Verification items for the finished model (mm, model axes). Face numbers are marked on the shaded views. A direction names the side the tool comes from. Round coordinates to 2 decimals unless told otherwise and drop trailing zeros. Write each loop counter-clockwise with the first axis right and the second up, starting at its lowest first coordinate (ties: lowest second). Pieces come first, ordered by that corner, then holes.
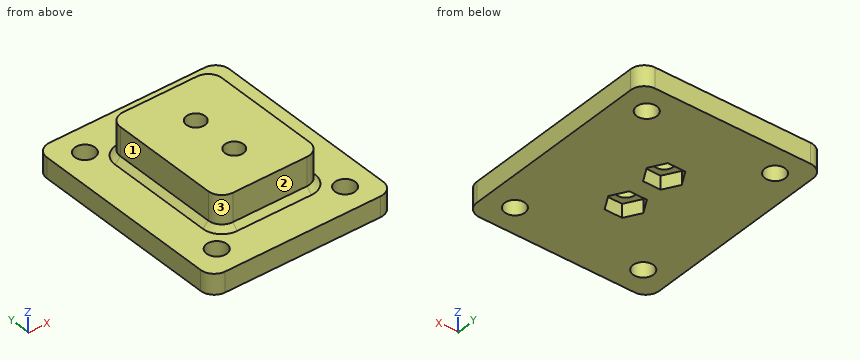
from build123d import *

# Parameters (mm, degrees)
F0_R     = 4.365625
F0_R_2   = 4.7625
F1_DEPTH = 9.525
F2_DEPTH = 25.4
F3_SIZE  = 2.54
F4_DEPTH = 6.35


with BuildPart() as f1:
    # F0 (on Top) → F1 (new body)
    with BuildSketch(Plane.XY):
        Polygon((-4.124446, -18.25625), (4.124446, -18.25625), (8.248892, -11.1125), (4.124446, -3.96875), (-4.124446, -3.96875), (-8.248892, -11.1125), align=None)
        with Locations((0, -11.1125)):
            Circle(F0_R, mode=Mode.SUBTRACT)
        with BuildLine():
            Line((17.4625, 31.75), (-17.4625, 31.75))
            ThreePointArc((-17.4625, 31.75), (-21.952628, 29.890128), (-23.8125, 25.4))
            Line((-23.8125, 25.4), (-23.8125, -25.4))
            ThreePointArc((-23.8125, -25.4), (-21.952628, -29.890128), (-17.4625, -31.75))
            Line((-17.4625, -31.75), (17.4625, -31.75))
            ThreePointArc((17.4625, -31.75), (21.952628, -29.890128), (23.8125, -25.4))
            Line((23.8125, -25.4), (23.8125, 25.4))
            ThreePointArc((23.8125, 25.4), (21.952628, 29.890128), (17.4625, 31.75))
        make_face()
        Polygon((8.248892, -11.1125), (4.124446, -18.25625), (-4.124446, -18.25625), (-8.248892, -11.1125), (-4.124446, -3.96875), (4.124446, -3.96875), align=None, mode=Mode.SUBTRACT)
        Polygon((-8.248892, 11.1125), (-4.124446, 18.25625), (4.124446, 18.25625), (8.248892, 11.1125), (4.124446, 3.96875), (-4.124446, 3.96875), align=None, mode=Mode.SUBTRACT)
        with BuildLine():
            Line((36.5125, 50.8), (-36.5125, 50.8))
            ThreePointArc((-36.5125, 50.8), (-41.002628, 48.940128), (-42.8625, 44.45))
            Line((-42.8625, 44.45), (-42.8625, -44.45))
            ThreePointArc((-42.8625, -44.45), (-41.002628, -48.940128), (-36.5125, -50.8))
            Line((-36.5125, -50.8), (36.5125, -50.8))
            ThreePointArc((36.5125, -50.8), (41.002628, -48.940128), (42.8625, -44.45))
            Line((42.8625, -44.45), (42.8625, 44.45))
            ThreePointArc((42.8625, 44.45), (41.002628, 48.940128), (36.5125, 50.8))
        make_face()
        with Locations((-30.1625, -38.1)):
            Circle(F0_R_2, mode=Mode.SUBTRACT)
        with Locations((30.1625, -38.1)):
            Circle(F0_R_2, mode=Mode.SUBTRACT)
        with BuildLine():
            ThreePointArc((-23.8125, 25.4), (-21.952628, 29.890128), (-17.4625, 31.75))
            Line((-17.4625, 31.75), (17.4625, 31.75))
            ThreePointArc((17.4625, 31.75), (21.952628, 29.890128), (23.8125, 25.4))
            Line((23.8125, 25.4), (23.8125, -25.4))
            ThreePointArc((23.8125, -25.4), (21.952628, -29.890128), (17.4625, -31.75))
            Line((17.4625, -31.75), (-17.4625, -31.75))
            ThreePointArc((-17.4625, -31.75), (-21.952628, -29.890128), (-23.8125, -25.4))
            Line((-23.8125, -25.4), (-23.8125, 25.4))
        make_face(mode=Mode.SUBTRACT)
        with Locations((-30.1625, 38.1)):
            Circle(F0_R_2, mode=Mode.SUBTRACT)
        with Locations((30.1625, 38.1)):
            Circle(F0_R_2, mode=Mode.SUBTRACT)
        Polygon((4.124446, 18.25625), (-4.124446, 18.25625), (-8.248892, 11.1125), (-4.124446, 3.96875), (4.124446, 3.96875), (8.248892, 11.1125), align=None)
        with Locations((0, 11.1125)):
            Circle(F0_R, mode=Mode.SUBTRACT)
    extrude(amount=F1_DEPTH)

    # F0 (on Top) → F2 (join)
    with BuildSketch(Plane.XY):
        with BuildLine():
            Line((17.4625, 31.75), (-17.4625, 31.75))
            ThreePointArc((-17.4625, 31.75), (-21.952628, 29.890128), (-23.8125, 25.4))
            Line((-23.8125, 25.4), (-23.8125, -25.4))
            ThreePointArc((-23.8125, -25.4), (-21.952628, -29.890128), (-17.4625, -31.75))
            Line((-17.4625, -31.75), (17.4625, -31.75))
            ThreePointArc((17.4625, -31.75), (21.952628, -29.890128), (23.8125, -25.4))
            Line((23.8125, -25.4), (23.8125, 25.4))
            ThreePointArc((23.8125, 25.4), (21.952628, 29.890128), (17.4625, 31.75))
        make_face()
        Polygon((8.248892, -11.1125), (4.124446, -18.25625), (-4.124446, -18.25625), (-8.248892, -11.1125), (-4.124446, -3.96875), (4.124446, -3.96875), align=None, mode=Mode.SUBTRACT)
        Polygon((-8.248892, 11.1125), (-4.124446, 18.25625), (4.124446, 18.25625), (8.248892, 11.1125), (4.124446, 3.96875), (-4.124446, 3.96875), align=None, mode=Mode.SUBTRACT)
        Polygon((4.124446, 18.25625), (-4.124446, 18.25625), (-8.248892, 11.1125), (-4.124446, 3.96875), (4.124446, 3.96875), (8.248892, 11.1125), align=None)
        with Locations((0, 11.1125)):
            Circle(F0_R, mode=Mode.SUBTRACT)
        Polygon((-4.124446, -18.25625), (4.124446, -18.25625), (8.248892, -11.1125), (4.124446, -3.96875), (-4.124446, -3.96875), (-8.248892, -11.1125), align=None)
        with Locations((0, -11.1125)):
            Circle(F0_R, mode=Mode.SUBTRACT)
    extrude(amount=F2_DEPTH)

    # F3
    f3_edges = [f1.edges().sort_by_distance(p)[0] for p in [
        (23.8125, 0, 9.525),
    ]]
    chamfer(f3_edges, length=F3_SIZE)

    # F0 (on Top) → F4 (cut)
    with BuildSketch(Plane.XY):
        Polygon((4.124446, 18.25625), (-4.124446, 18.25625), (-8.248892, 11.1125), (-4.124446, 3.96875), (4.124446, 3.96875), (8.248892, 11.1125), align=None)
        with Locations((0, 11.1125)):
            Circle(F0_R, mode=Mode.SUBTRACT)
        Polygon((-4.124446, -18.25625), (4.124446, -18.25625), (8.248892, -11.1125), (4.124446, -3.96875), (-4.124446, -3.96875), (-8.248892, -11.1125), align=None)
        with Locations((0, -11.1125)):
            Circle(F0_R, mode=Mode.SUBTRACT)
    extrude(amount=F4_DEPTH, mode=Mode.SUBTRACT)


solid = f1.part
Q1. Depth check by flat-ended pin: P1, Ø15, axis at x = -30.16, y = -38.1, coming from the +Z side (3 decimals); P2, Ø3, axis at y = -23, z = 13, coming from the -X side; P3, Ø12, axis at x = 13, z = 21.5, coming from the +Y side. Enter the tip coordinate at first touch or a pass-through.
Recorded:
P1: stops at z = 9.525
P2: stops at x = -24.38
P3: stops at y = 31.75
Q2. Material ranges on line 1 along Y through (x, z) = (2, 10.5) (3 decimals); line 2 along Y through (x, z) = (15, 20); line 3 along Z through (x, y) = (-20, 41.5) (3 decimals), recorded low to high.
Recorded:
line 1: y = -33.315 to -14.993, -7.232 to 7.232, 14.993 to 33.315
line 2: y = -31.75 to 31.75
line 3: z = 0 to 9.525
Q3. Sectioned sample at C-C (z = 2). Give the number of separate pieces and of enclosed holes in the cut face, plus the area to 3 significant figures.
Recorded:
separate pieces: 1
enclosed holes: 6
area: 8,040 mm2
Q4. Tool access check on the marked faces 1, 2 and 3. Record the directions out of +Z, -Z, +X, -X, +Y, -Y that give a thin tool (end or side, any length) a straight path to the whole face; none if there is none.
Recorded:
face 1: +Z, -X, +Y, -Y
face 2: +Z, +X, -X, -Y
face 3: +Z, -X, -Y
Q5. Sectioned sample at A-A (x = 0). Enter the section's corners in (y, z) (3 decimals), plus the area to 3 significant figures.
Recorded:
outline: (-50.8, 0) - (-18.256, 0) - (-18.256, 6.35) - (-15.478, 6.35) - (-15.478, 25.4) - (-31.75, 25.4) - (-31.75, 12.065) - (-34.29, 9.525) - (-50.8, 9.525) - close; (-6.747, 6.35) - (-3.969, 6.35) - (-3.969, 0) - (3.969, 0) - (3.969, 6.35) - (6.747, 6.35) - (6.747, 25.4) - (-6.747, 25.4) - close; (15.478, 6.35) - (18.256, 6.35) - (18.256, 0) - (50.8, 0) - (50.8, 9.525) - (34.29, 9.525) - (31.75, 12.065) - (31.75, 25.4) - (15.478, 25.4) - close
area: 1,470 mm2
Q6. Sectioned sample at B-B (y = -38.1). Enter the section's corners in (x, z) (1 decimal).
Recorded:
outline: (-42.9, 0) - (-34.9, 0) - (-34.9, 9.5) - (-42.9, 9.5) - close; (-25.4, 0) - (25.4, 0) - (25.4, 9.5) - (-25.4, 9.5) - close; (34.9, 0) - (42.9, 0) - (42.9, 9.5) - (34.9, 9.5) - close
Q7. Sectioned sample at D-D (z = 20). Enter the section's corners in (x, y), plus the area to 3 significant figures.
Recorded:
outline: (-23.81, -25.4) arc R6.35 ccw to (-17.46, -31.75) - (17.46, -31.75) arc R6.35 ccw to (23.81, -25.4) - (23.81, 25.4) arc R6.35 ccw to (17.46, 31.75) - (-17.46, 31.75) arc R6.35 ccw to (-23.81, 25.4) - close; hole circle Ø8.73 at (0, -11.11); hole circle Ø8.73 at (0, 11.11)
area: 2,870 mm2
